Geometry: final body of the model. Coordinates: model frame, mm. A direction names the side the tool comes from. Coordinates: 2 decimals unless noted, no trailing zeros. Write each loop counter-clockwise with the first axis right and the second up, starting at its lowest first coordinate (ties: lowest second). Pieces come first, ordered by that corner, then holes. Notation, with made-up numbers: (71, -35) -> (105, -35) arc R15 ccw to (105, -18) -> close; hole circle Ø3 at (16, 23.5). An arc over 180 degrees is marked (long way). One line per item, written item: value.
```python
from build123d import *

# Parameters (mm, degrees)
F0_R     = 38
F0_R_2   = 3
F1_DEPTH = 3
F2_DEPTH = 10
F0_R_3   = 40
F3_DEPTH = 5


with BuildPart() as f1:
    # F0 (on Top) → F1 (new body)
    with BuildSketch(Plane.XY):
        Circle(F0_R)
        with Locations((-15, -15)):
            Circle(F0_R_2, mode=Mode.SUBTRACT)
        with Locations((0, -15)):
            Circle(F0_R_2, mode=Mode.SUBTRACT)
        with Locations((15, -15)):
            Circle(F0_R_2, mode=Mode.SUBTRACT)
        with Locations((-15, 0)):
            Circle(F0_R_2, mode=Mode.SUBTRACT)
        with Locations((-15, 15)):
            Circle(F0_R_2, mode=Mode.SUBTRACT)
        Circle(F0_R_2, mode=Mode.SUBTRACT)
        with Locations((15, 0)):
            Circle(F0_R_2, mode=Mode.SUBTRACT)
        with Locations((0, 15)):
            Circle(F0_R_2, mode=Mode.SUBTRACT)
        with Locations((15, 15)):
            Circle(F0_R_2, mode=Mode.SUBTRACT)
    extrude(amount=F1_DEPTH)

    # F0 (on Top) → F2 (join)
    with BuildSketch(Plane.XY):
        with Locations((0, 15)):
            Circle(F0_R_2)
        with Locations((-15, 0)):
            Circle(F0_R_2)
        with Locations((0, -15)):
            Circle(F0_R_2)
        with Locations((15, 0)):
            Circle(F0_R_2)
        with Locations((-15, 15)):
            Circle(F0_R_2)
        with Locations((15, 15)):
            Circle(F0_R_2)
        with Locations((15, -15)):
            Circle(F0_R_2)
        Circle(F0_R_2)
        with Locations((-15, -15)):
            Circle(F0_R_2)
    extrude(amount=F2_DEPTH)

    # F0 (on Top) → F3 (join)
    with BuildSketch(Plane.XY):
        Circle(F0_R_3)
        Circle(F0_R, mode=Mode.SUBTRACT)
    extrude(amount=F3_DEPTH)


solid = f1.part
```
(1) First-contact query: pin 1 (1 mm diameter, centred on x = 26, y = -10, fed in from -Z); pin 2 (1 mm diameter, centred on x = -17, y = -31, fed in from +Z); pin 3 (6 mm diameter, centred on y = -14, z = 2.5, fed in from -X); pin 4 (1 mm diameter, centred on x = -2.5, z = 3, fed in from +Y). Flat tips, straight axial feed; report the tip coordinate or a pass-through.
Responses:
pin 1: stops at z = 0
pin 2: stops at z = 3
pin 3: stops at x = -38.46
pin 4: stops at y = 39.95
(2) Pull-direction query (X, two-part tool) for faces 1 (the cylindrical face through (-8.67, -39.05, 2.46)), 2 (the flat face through (35.4, -14.6, 5)), 3 (the cylindrical face through (-3, 0, 6)); classes: released by +X, released by -X, zero draft, split by the parting line, or undercut.
Responses:
face 1: split by the parting line
face 2: zero draft
face 3: undercut
(3) Section D-D (x = 24). Return the cut outline in (y, z), then the cut area to 3 significant figures.
Responses:
outline: (-32, 0) -> (32, 0) -> (32, 5) -> (29.46, 5) -> (29.46, 3) -> (-29.46, 3) -> (-29.46, 5) -> (-32, 5) -> close
area: 202 mm2
(4) Line query: line 1 (Y direction, x = 0, z = 8.75); line 2 (Y direction, x = 0, z = 3.6); line 3 (Y direction, x = 2, z = 6). Output: solid intervals per line, ascending. Write a range as [from, to].
Responses:
line 1: y = [-18, -12], [-3, 3], [12, 18]
line 2: y = [-40, -38], [-18, -12], [-3, 3], [12, 18], [38, 40]
line 3: y = [-17.24, -12.76], [-2.24, 2.24], [12.76, 17.24]
(5) Section B-B (y = -21). Return the cut outline in (x, z), then the cut area to 3 significant figures.
Responses:
outline: (-34.04, 0) -> (34.04, 0) -> (34.04, 5) -> (31.67, 5) -> (31.67, 3) -> (-31.67, 3) -> (-31.67, 5) -> (-34.04, 5) -> close
area: 214 mm2
(6) Section A-A (x = 0). Return the cut outline in (y, z), then the cut area to 3 significant figures.
Responses:
outline: (-40, 0) -> (40, 0) -> (40, 5) -> (38, 5) -> (38, 3) -> (18, 3) -> (18, 10) -> (12, 10) -> (12, 3) -> (3, 3) -> (3, 10) -> (-3, 10) -> (-3, 3) -> (-12, 3) -> (-12, 10) -> (-18, 10) -> (-18, 3) -> (-38, 3) -> (-38, 5) -> (-40, 5) -> close
area: 374 mm2
(7) Reachability of faces 4 (the flat face through (0, 0, 10)), 5 (the cylindrical face through (-17.4, -16.8, 6.5)) from +Z, -Z, +X, -X, +Y, -Y: full face, straight path, thin tool, end or side. Return the list, or none.
Responses:
face 4: +Z, +X, -X, +Y, -Y
face 5: +Z
(8) Section C-C (z = 2). Return the cut outline in (x, y).
Responses:
outline: circle Ø80 at (0, 0)
